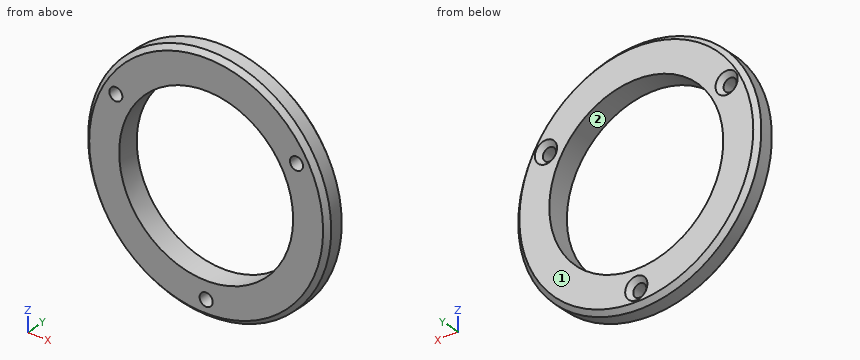
from build123d import *

# Parameters (mm, degrees)
SKETCH1_R           = 26.543
SKETCH1_R_2         = 19
SKETCH1_R_3         = 1.425
BOSS_EXTRUDE1_DEPTH = 5
CHAMFER1_SIZE       = 1
CHAMFER2_SIZE       = 1
CHAMFER3_SIZE       = 1
CHAMFER4_SIZE       = 1
CHAMFER5_SIZE       = 1


with BuildPart() as part:
    # Sketch1 → Boss-Extrude1 (new body)
    with BuildSketch(Plane(origin=(0, 0, 0), x_dir=(1, 0, 0), z_dir=(0, 1, 0))):
        Circle(SKETCH1_R)
        Circle(SKETCH1_R_2, mode=Mode.SUBTRACT)
        with Locations((0, 22.776724903)):
            Circle(SKETCH1_R_3, mode=Mode.SUBTRACT)
        with Locations((19.725222381, -11.388362451)):
            Circle(SKETCH1_R_3, mode=Mode.SUBTRACT)
        with Locations((-19.725222381, -11.388362451)):
            Circle(SKETCH1_R_3, mode=Mode.SUBTRACT)
    extrude(amount=BOSS_EXTRUDE1_DEPTH)

    # Chamfer1
    chamfer1_edges = [part.edges().sort_by_distance(p)[0] for p in [
        (-1.425, 5, -22.776724903),
    ]]
    chamfer(chamfer1_edges, length=CHAMFER1_SIZE)

    # Chamfer2
    chamfer2_edges = [part.edges().sort_by_distance(p)[0] for p in [
        (-21.150222381, 5, 11.388362451),
    ]]
    chamfer(chamfer2_edges, length=CHAMFER2_SIZE)

    # Chamfer3
    chamfer3_edges = [part.edges().sort_by_distance(p)[0] for p in [
        (18.300222381, 5, 11.388362451),
    ]]
    chamfer(chamfer3_edges, length=CHAMFER3_SIZE)

    # Chamfer4
    chamfer4_edges = [part.edges().sort_by_distance(p)[0] for p in [
        (-26.543, 5, 0),
    ]]
    chamfer(chamfer4_edges, length=CHAMFER4_SIZE)

    # Chamfer5
    chamfer5_edges = [part.edges().sort_by_distance(p)[0] for p in [
        (-26.543, 0, 0),
    ]]
    chamfer(chamfer5_edges, length=CHAMFER5_SIZE)


solid = part.part
Geometry check sheet. Reference: the model listing, model coordinates, mm. Face numbers are marked on the shaded views. Round coordinates to 2 decimals unless told otherwise and drop trailing zeros. Write each loop counter-clockwise with the first axis right and the second up, starting at its lowest first coordinate (ties: lowest second). Pieces come first, ordered by that corner, then holes. Notation, with made-up numbers: (-26, 44.5) -> (30, 44.5) arc R21 ccw to (30, 78.5) -> close; hole circle Ø11 at (-30, 23). An arc over 180 degrees is marked (long way). One line per item, written item: value. Start each with the question number.
(1) Cross-section at A-A, the plane x = 0. Record the cut outline in (y, z).
(2) Scan lines: line 1 (X direction, y = 2.95, z = 0.5); line 2 (Z direction, x = -8, y = 4.75); line 3 (Z direction, x = -11.5, y = 4.3). Record each from-to range of solid material in increasing order. Write a range as [from, to].
(3) Cross-section at C-C, the plane y = 1.7. Record the cut outline in (x, z) (3 decimals).
(4) Go/stop test with flat-tipped pins: pin 1 Ø3 at (x, y) = (-5.5, 4) entering from +Z; pin 2 Ø23 at (x, z) = (0, 0) entering from -Y; pin 3 Ø4.5 at (x, z) = (-19.73, 11.39) entering from +Y; pin 4 Ø1.5 at (y, z) = (1.5, -15.5) entering from -X. Record where each tip stops, or that it passes through.
(5) Draft check along Z on the marked faces 1 and 2. Enter one of: +Z half, -Z half, draft (parallel to the pull), parting line (faces both ways), or undercut.
(6) Cross-section at B-B, the plane z = 0. Record the cut outline in (x, y).
Answer:
1. outline: (0, -25.54) -> (1, -26.54) -> (4, -26.54) -> (5, -25.54) -> (5, -25.2) -> (4, -24.2) -> (0, -24.2) -> close; (0, -21.35) -> (4, -21.35) -> (5, -20.35) -> (5, -19) -> (0, -19) -> close; (0, 19) -> (5, 19) -> (5, 25.54) -> (4, 26.54) -> (1, 26.54) -> (0, 25.54) -> close
2. line 1: [-26.54, -18.99], [18.99, 26.54]
2. line 2: [-24.52, -17.23], [17.23, 24.52]
2. line 3: [-23.59, -15.12], [15.12, 23.59]
3. outline: circle Ø53.086 at (0, 0); hole circle Ø2.85 at (-19.725, 11.388); hole circle Ø38 at (0, 0); hole circle Ø2.85 at (0, -22.777); hole circle Ø2.85 at (19.725, 11.388)
4. pin 1: z = 26.24
4. pin 2: through
4. pin 3: y = 4.83
4. pin 4: x = -22.07
5. face 1: draft
5. face 2: undercut
6. outline: (-26.54, 1) -> (-25.54, 0) -> (-19, 0) -> (-19, 5) -> (-25.54, 5) -> (-26.54, 4) -> close; (19, 0) -> (25.54, 0) -> (26.54, 1) -> (26.54, 4) -> (25.54, 5) -> (19, 5) -> close
